Source: CAD feature listing. Evaluate the final solid. Frame: model axes, mm. A direction names the side the tool comes from. Give positions to 0.01 mm unless a question says otherwise; leave off trailing zeros. Order: outer loops, then holes, each group sorted by start corner. A loop starts at its lowest first (then second) coordinate and runs counter-clockwise, first axis right, second up. Notation, with made-up numbers: M 5,-27 L 11,-27 A17 cw 11,-3 Z; hole C -10.75,-30 d9. An arc over 180 degrees is marked long. One line per question, with ' | ' between items. Start each with the question number.
from build123d import *

# Parameters (mm, degrees)
EXTRUDE_DEPTH   = 79
POCKET_DEPTH    = 6
POCKET001_DEPTH = 6


with BuildPart() as obj1:
    # Part__Mirroring → Extrude (new body)
    with BuildSketch(Plane(origin=(-25, -1.004737, 0), x_dir=(0, 1, 0), z_dir=(0, 0, 1))):
        with BuildLine():
            ThreePointArc((14.004737, -25), (11.372036, -17.156587), (4.540257, -12.49))
            Line((4.540257, -12.49), (-4.000791, -5))
            Line((-4.000791, -5), (-4.004737, 25))
            Line((-4.004737, 25), (-14.004737, 25))
            Line((-14.004737, 25), (-14.004737, -25))
            Line((-14.004737, -25), (-2.745263, -25))
            ThreePointArc((-2.745263, -25), (1.004737, -21.25), (4.754737, -25))
            Line((4.754737, -25), (14.004737, -25))
        make_face()
    extrude(amount=EXTRUDE_DEPTH)


with BuildPart() as body001:
    # Part__Mirroring001: instance of obj1
    add(obj1.part.mirror(Plane(origin=(0, 0, 0), x_dir=(0, -1, 0), z_dir=(1, 0, 0))))

    # Fusion: union obj1
    add(obj1.part)

    # Sketch001 → Pocket (cut)
    with BuildSketch(Plane.XY):
        Polygon((0, -7.5), (6.495191, -3.75), (6.495191, 3.75), (0, 7.5), (-6.495191, 3.75), (-6.495191, -3.75), align=None)
    extrude(amount=POCKET_DEPTH, mode=Mode.SUBTRACT)

    # Sketch002 (on Face5 of Pocket) → Pocket001 (cut)
    with BuildSketch(Plane.XY.offset(79)):
        Polygon((0, -7.5), (6.495191, -3.75), (6.495191, 3.75), (0, 7.5), (-6.495191, 3.75), (-6.495191, -3.75), align=None)
    extrude(amount=-POCKET001_DEPTH, mode=Mode.SUBTRACT)


solid = body001.part
Item 1: Cut plane C-C on y = 6.25. Return the cut outline in (x, z).
Item 2: Mould query, pull axis Y, two halves, no side actions, for faces 1 (the flat face through (50, -10, 39)), 2 (the flat face through (-1, -15.009, 39)), 3 (the flat face through (3.202, -5.651, 76.042)), 4 (the flat face through (3.29, 5.6, 2.96)). Classes: pulls with the +Y half, pulls with the -Y half, needs draft (parallel to the pull), parting line crosses it, or undercut.
Item 3: Cut plane D-D on x = -33. Return the cut outline in (y, z).
Item 4: Cut plane A-A on z = 67.5. Return the cut outline in (x, y), and give its area (3 significant figures).
Item 5: Pin query (flat end, axial travel): pin 1 Ø4 at (x, y) = (1, -1) entering from +Z; pin 2 Ø12 at (x, z) = (9, 26.5) entering from +Y; pin 3 Ø5 at (x, z) = (-10, 56.5) entering from +Y; pin 4 Ø10 at (y, z) = (3, 65) entering from +X. Return the tip coordinate at first contact, or that it passes through.
Item 6: Cut plane B-B on y = 0. Return the cut outline in (x, z).
Item 7: Reachability of faces 5 (the flat face through (-0.7, -7.4, 79)), 6 (the flat face through (-6.495, 0, 3)), 7 (the flat face through (-3, -3, 73)) from +Z, -Z, +X, -X, +Y, -Y: full face, straight path, thin tool, end or side. Return the list, or none.
Item 8: Line query: line 1 (Y direction, x = -30.5, z = 27); line 2 (Y direction, x = -5, z = 4.5); line 3 (X direction, y = -0.5, z = 61.5). Output: solid intervals per line, ascending.
Results are:
1) outline: M -11.4,0 L -2.17,0 L -2.17,6 L 2.17,6 L 2.17,0 L 11.4,0 L 11.4,79 L 2.17,79 L 2.17,73 L -2.17,73 L -2.17,79 L -11.4,79 Z
2) face 1: needs draft | face 2: pulls with the -Y half | face 3: undercut | face 4: undercut
3) outline: M -15.01,0 L -5.01,0 L -5.01,79 L -15.01,79 Z
4) outline: M -50,-15.01 L 50,-15.01 L 50,-5.01 L 20,-5.01 L 12.51,3.54 A13 ccw 0,13 A13 ccw -12.51,3.54 L -20,-5.01 L -50,-5.01 Z; hole C 0,0 d7.5 | area: 1,410 mm2
5) pin 1: passes through | pin 2: stops at y = 12.65 | pin 3: stops at y = 10.62 | pin 4: stops at x = 17.36
6) outline: M -15.61,0 L -6.5,0 L -6.5,6 L -3.75,6 L -3.75,73 L -6.5,73 L -6.5,79 L -15.61,79 Z; M 3.75,6 L 6.5,6 L 6.5,0 L 15.61,0 L 15.61,79 L 6.5,79 L 6.5,73 L 3.75,73 Z
7) face 5: +Z, +X, -X, +Y, -Y | face 6: -Z | face 7: +Z
8) line 1: y = -15.01 to -5.01 | line 2: y = -15.01 to -4.61, 4.61 to 12 | line 3: x = -16.05 to -3.72, 3.72 to 16.05
